Work out the finished part from the listing and answer in its coordinate system (mm). Face numbers are marked on the shaded views. A direction names the side the tool comes from. Give positions to 0.01 mm unless a question says otherwise; leave off trailing zeros. Write each loop counter-clockwise with the first axis right and the second up, starting at its lowest first coordinate (ties: lowest second). Pieces come first, ordered by that corner, then holes. Notation, with made-up numbers: (8, -30.5) - (42, -30.5) arc R22 ccw to (42, -6.5) - close; hole circle Ø7 at (-1, 43). An arc over 180 degrees is marked (long way). Write item = value, one per line.
from build123d import *

# Parameters (mm, degrees)
SKETCH_1_W      = 4
SKETCH_1_H      = 4
EXTRUDE_1_DEPTH = 16
SKETCH_3_R      = 1
EXTRUDE_2_DEPTH = 8


with BuildPart() as part:
    # 草图1 → 凸台-拉伸1 (new body)
    with BuildSketch(Plane.XY):
        Rectangle(SKETCH_1_W, SKETCH_1_H)
    extrude(amount=EXTRUDE_1_DEPTH)

    # 草图3 → 凸台-拉伸2 (add, symmetric)
    with BuildSketch(Plane(origin=(0, 0, 0), x_dir=(1, 0, 0), z_dir=(0, 1, 0))):
        with Locations((1, 0)):
            Circle(SKETCH_3_R)
    extrude(amount=EXTRUDE_2_DEPTH, both=True)


solid = part.part
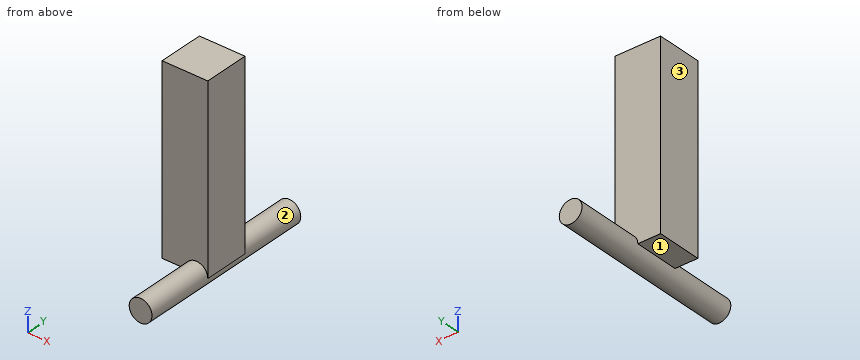
1. Find section D-D, the plane x = -1.1. Give the vertices of the cut face in (y, z).
Solution:
outline = (-2, 0) - (2, 0) - (2, 16) - (-2, 16) - close
2. Find section B-B, the plane y = -1.5. Give the vertices of the cut face in (x, z).
Solution:
outline = (-2, 0) - (0, 0) arc R1 ccw to (2, 0) - (2, 16) - (-2, 16) - close
3. Find section A-A, the plane x = 1. Give the vertices of the cut face in (y, z).
Solution:
outline = (-8, -1) - (8, -1) - (8, 1) - (2, 1) - (2, 16) - (-2, 16) - (-2, 1) - (-8, 1) - close
4. Straight lines are drawn through the part: line 1 (Z direction, x = 1.05, y = 6); line 2 (Y direction, x = -1.3, z = 7.25); line 3 (X direction, y = -6, z = 0). For each, find the intervals that lie inside material, in ascending order.
Solution:
line_1 = -1 to 1
line_2 = -2 to 2
line_3 = 0 to 2
5. Find section C-C, the plane z = 10.75. Give the vertices of the cut face in (x, y).
Solution:
outline = (-2, -2) - (2, -2) - (2, 2) - (-2, 2) - close
6. A tool of negligible diameter and unlimited length cuts with its end or side. For the marked faces 1, 2 and 3, from which of +Z, -Z, +X, -X, +Y, -Y can it reach the whole face along a straight path? Write none if from no direction.
Solution:
face_1 = -Z, -X, +Y, -Y
face_2 = none
face_3 = +Z, -Z, -X, +Y, -Y
7. Given pin 1 (5 mm diameter, centred on y = -3, z = 9.5, fed in from +X); pin 2 (2 mm diameter, centred on x = -1.5, y = 0.5, fed in from -Z); pin 3 (2 mm diameter, centred on x = 0.5, z = 7, fed in from +Y); pin 4 (1 mm diameter, centred on x = -1, z = 10.5, fed in from -Y), each flat-ended and moving along its own axis, determine where each tip first touches the part or whether it passes through.
Solution:
pin_1 = 2
pin_2 = 0
pin_3 = 2
pin_4 = -2
